```python
from build123d import *

# Parameters (mm, degrees)
SKETCH1_W   = 127
SKETCH1_H   = 76.2
BASE_DEPTH  = 9.525
SKETCH2_R   = 4.7625
HOLES_DEPTH = 149.412147835
FILLET2_R   = 1.5875


with BuildPart() as part:
    # Sketch1 → base (new body)
    with BuildSketch(Plane.XY):
        with Locations((63.5, 38.1)):
            Rectangle(SKETCH1_W, SKETCH1_H)
    extrude(amount=BASE_DEPTH)

    # Sketch2 → holes (cut, through all)
    with BuildSketch(Plane.XY):
        with Locations((15.875, 15.875)):
            Circle(SKETCH2_R)
        with Locations((111.125, 15.875)):
            Circle(SKETCH2_R)
        with Locations((15.875, 60.325)):
            Circle(SKETCH2_R)
        with Locations((111.125, 60.325)):
            Circle(SKETCH2_R)
    extrude(amount=HOLES_DEPTH, mode=Mode.SUBTRACT)

    # Fillet2
    fillet2_edges = [part.edges().sort_by_distance(p)[0] for p in [
        (63.5, 76.2, 9.525),
    ]]
    fillet(fillet2_edges, radius=FILLET2_R)


solid = part.part
```
Part model, mm, in its own coordinate system. Round coordinates to 2 decimals unless told otherwise and drop trailing zeros. Loops run counter-clockwise (first coordinate to the right, second up) from the corner with the lowest first, then second, coordinate; pieces in that order, holes last.
Item 1: Cut at B-B, the plane x = 109.5. Give the cut face in (y, z) (1 decimal).
Item 2: Drill centre lines: line 1 (Y direction, x = 15.5, z = 1.5); line 2 (X direction, y = 12, z = 8.25); line 3 (Y direction, x = 14, z = 0.75). Where is each one in solid material? Low to high.
Item 3: Cut at C-C, the plane z = 5.75. Give the cut face in (x, y) (1 decimal).
Item 4: Drop a flat-ended pin along its axis: P1, Ø5.5, axis at x = 15.875, y = 60.325, coming from the +Z side (3 decimals). Give the stop position or say it passes through.
Item 5: Cut at A-A, the plane y = 14. Give the cut face in (x, z) (3 decimals), then the cut area to 3 significant figures.
Item 6: Mould opens along Y. For faces 1 (the face through (63, 0, 5)), 2 (the face through (106.367, 60.534, 4.696)), 3 (the face through (63, 39, 0)) say: +Y half, -Y half, draft (parallel to the pull), parting line (faces both ways), or undercut.
Item 7: Cut at D-D, the plane y = 57. Give the cut face in (x, z) (3 decimals).
A:
1. outline: (0, 0) - (11.4, 0) - (11.4, 9.5) - (0, 9.5) - close; (20.4, 0) - (55.8, 0) - (55.8, 9.5) - (20.4, 9.5) - close; (64.8, 0) - (76.2, 0) - (76.2, 7.9) arc R1.6 ccw to (74.6, 9.5) - (64.8, 9.5) - close
2. line 1: y = 0 to 11.13, 20.62 to 55.58, 65.07 to 76.2
2. line 2: x = 0 to 13.11, 18.64 to 108.36, 113.89 to 127
2. line 3: y = 0 to 11.5, 20.25 to 55.95, 64.7 to 76.2
3. outline: (0, 0) - (127, 0) - (127, 76.2) - (0, 76.2) - close; hole circle Ø9.5 at (15.9, 15.9); hole circle Ø9.5 at (15.9, 60.3); hole circle Ø9.5 at (111.1, 15.9); hole circle Ø9.5 at (111.1, 60.3)
4. P1: passes through
5. outline: (0, 0) - (11.497, 0) - (11.497, 9.525) - (0, 9.525) - close; (20.253, 0) - (106.747, 0) - (106.747, 9.525) - (20.253, 9.525) - close; (115.503, 0) - (127, 0) - (127, 9.525) - (115.503, 9.525) - close
5. area: 1,040 mm2
6. face 1: -Y half
6. face 2: undercut
6. face 3: draft
7. outline: (0, 0) - (12.465, 0) - (12.465, 9.525) - (0, 9.525) - close; (19.285, 0) - (107.715, 0) - (107.715, 9.525) - (19.285, 9.525) - close; (114.535, 0) - (127, 0) - (127, 9.525) - (114.535, 9.525) - close
